Study the drawing (mm; zero at the part's minimum x, y, z) and answer. A direction names the side the tool comes from. Coordinates: 2 decimals unless noted, no trailing zeros. Order: outer loops, then holes, each group sorted by start corner. A loop starts at its lowest first (then second) coordinate and runs counter-clockwise, first axis right, second up. Notation, with made-up numbers: M -27.75,-4.75 L -13.75,-4.75 A16 ccw -13.75,24.25 Z; hole C 50.25,64.5 d6. An arc over 180 degrees is marked long. One line per item, written item: value. Start each with the question number.
Q1. The part is cut by section B-B on x = 67. Give the vertices of the cut face in (y, z) (1 decimal), then the cut area to 3 significant figures.
Q2. For the marked faces 4, 5 and 6, determine the directions among +Z, -Z, +X, -X, +Y, -Y from which every point of the face is accessible in a straight line to the end or side of a thin tool.
Q3. The part is cut by section D-D on x = 38. Give the vertices of the cut face in (y, z), then the cut area to 3 significant figures.
Q4. The part is cut by section A-A on y = 67. Give the vertices of the cut face in (x, z) (1 decimal).
Q5. Each of these flat-tipped pins is pushed along its axis until it touches: pin 1 Ø5 at (y, z) = (6.5, 4.5) entering from +X; pin 2 Ø5 at (x, z) = (55, 8) entering from +Y; pin 3 Ø6 at (x, z) = (66, 5) entering from -Y; pin 4 Ø2 at (x, y) = (61.5, 53) entering from +Z. Where does it stop, or does it pass through?
Q6. Straight lines are drawn through the part: line 1 along X through (y, z) = (62, 3) (1 decimal); line 2 along Z through (x, y) = (43.5, 67); line 3 along Y through (x, z) = (61, 10.75) (1 decimal). For each, find the intervals that lie inside material, in ascending order. Write a range as [from, to].
Q7. The part is cut by section C-C on z = 10.5. Give the vertices of the cut face in (x, y) (1 decimal), then the cut area to 3 significant figures.
Q8. Determine the mould class of the marked faces 1, 2 and 3 for opening direction X: pulls with the +X half, pulls with the -X half, needs draft (parallel to the pull), parting line crosses it, or undercut.
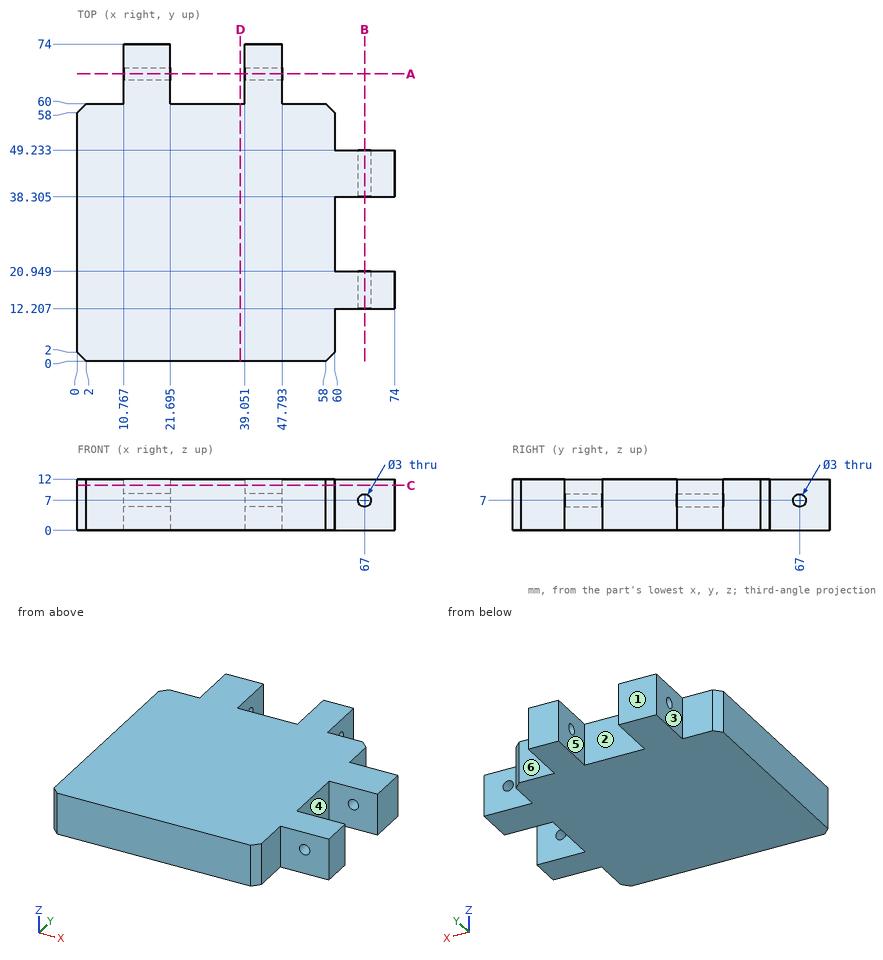
Output:
1. outline: M 12.2,0 L 20.9,0 L 20.9,5.5 L 12.2,5.5 Z; M 12.2,8.5 L 20.9,8.5 L 20.9,12 L 12.2,12 Z; M 38.3,0 L 49.2,0 L 49.2,5.5 L 38.3,5.5 Z; M 38.3,8.5 L 49.2,8.5 L 49.2,12 L 38.3,12 Z
1. area: 177 mm^2
2. face 4: +Z, -Z, +X
2. face 5: +Z, -Z, +Y
2. face 6: +Z, -Z, +X, +Y
3. outline: M 0,0 L 60,0 L 60,12 L 0,12 Z
3. area: 720 mm^2
4. outline: M 10.8,0 L 21.7,0 L 21.7,5.5 L 10.8,5.5 Z; M 10.8,8.5 L 21.7,8.5 L 21.7,12 L 10.8,12 Z; M 39.1,0 L 47.8,0 L 47.8,5.5 L 39.1,5.5 Z; M 39.1,8.5 L 47.8,8.5 L 47.8,12 L 39.1,12 Z
5. pin 1: stops at x = 60
5. pin 2: stops at y = 60
5. pin 3: stops at y = 12.21
5. pin 4: passes through
6. line 1: x = [10.8, 21.7], [39.1, 47.8]
6. line 2: z = [0, 5.5], [8.5, 12]
6. line 3: y = [12.2, 20.9], [38.3, 49.2]
7. outline: M 0,2 L 2,0 L 58,0 L 60,2 L 60,12.2 L 74,12.2 L 74,20.9 L 60,20.9 L 60,38.3 L 74,38.3 L 74,49.2 L 60,49.2 L 60,58 L 58,60 L 47.8,60 L 47.8,74 L 39.1,74 L 39.1,60 L 21.7,60 L 21.7,74 L 10.8,74 L 10.8,60 L 2,60 L 0,58 Z
7. area: 4,140 mm^2
8. face 1: needs draft
8. face 2: undercut
8. face 3: pulls with the -X half
